from build123d import *

# Parameters (mm, degrees)
PAD_DEPTH       = 40
POCKET_DEPTH    = 35
FILLET_R        = 2
SKETCH002_R     = 1.75
POCKET001_DEPTH = 40.001


with BuildPart() as part:
    # Sketch → Pad (new body)
    with BuildSketch(Plane.XY):
        with BuildLine():
            ThreePointArc((14.201108, 23.840953), (-0.00078, 27.75), (-14.202448, 23.840154))
            ThreePointArc((-14.202448, 23.840154), (-14.967616, 21.462867), (-13.949732, 19.182322))
            ThreePointArc((-19.182322, 13.949732), (-13.949732, 13.949732), (-13.949732, 19.182322))
            ThreePointArc((-19.182322, 13.949732), (-21.992232, 14.881289), (-24.417911, 13.184389))
            ThreePointArc((-24.417911, 13.184389), (-27.743827, -0.585306), (-23.840136, -14.202479))
            ThreePointArc((-23.840136, -14.202479), (-21.462853, -14.967618), (-19.182322, -13.949732))
            ThreePointArc((-13.949732, -13.949732), (-16.566027, -12.866027), (-19.182322, -13.949732))
            ThreePointArc((-13.949732, -13.949732), (0, -19.7279), (13.949732, -13.949732))
            ThreePointArc((19.182322, -13.949732), (16.566027, -12.866027), (13.949732, -13.949732))
            ThreePointArc((19.182322, -13.949732), (21.462854, -14.967618), (23.840137, -14.202477))
            ThreePointArc((23.840137, -14.202477), (27.75, -4.3e-05), (23.840181, 14.202403))
            ThreePointArc((23.840181, 14.202403), (21.462879, 14.967595), (19.182307, 13.949717))
            ThreePointArc((13.934503, 19.167004), (13.957373, 13.942113), (19.182307, 13.949717))
            ThreePointArc((13.934503, 19.167004), (14.950896, 21.453606), (14.201108, 23.840953))
        make_face()
    extrude(amount=PAD_DEPTH)

    # Sketch001 (on Face15 of Pad) → Pocket (cut)
    with BuildSketch(Plane(origin=(0, 0, 0), x_dir=(1, 0, 0), z_dir=(0, 0, -1))):
        with BuildLine():
            ThreePointArc((-21.578938, 12.120723), (-16.766795, 9.869036), (-11.828409, 11.828414))
            ThreePointArc((11.828412, 11.828411), (2e-06, 16.7279), (-11.828409, 11.828414))
            ThreePointArc((11.828412, 11.828411), (16.766797, 9.869036), (21.578938, 12.120723))
            ThreePointArc((21.578938, -12.120723), (24.75, 0), (21.578938, 12.120723))
            ThreePointArc((21.578938, -12.120723), (11.828412, -11.828412), (12.120723, -21.578938))
            ThreePointArc((-12.120723, -21.578938), (0, -24.75), (12.120723, -21.578938))
            ThreePointArc((-12.120723, -21.578938), (-11.828412, -11.828412), (-21.578938, -12.120723))
            ThreePointArc((-21.578938, 12.120723), (-24.75, 0), (-21.578938, -12.120723))
        make_face()
    extrude(amount=-POCKET_DEPTH, mode=Mode.SUBTRACT)

    # Fillet
    fillet_edges = [part.edges().sort_by_distance(p)[0] for p in [
        (-21.578938, 12.120723, 17.5),
        (-12.120723, 21.578938, 17.5),
        (12.120723, 21.578938, 17.5),
        (21.578938, 12.120723, 17.5),
        (21.578938, -12.120723, 17.5),
        (-21.578938, -12.120723, 17.5),
    ]]
    fillet(fillet_edges, radius=FILLET_R)

    # Sketch002 (on Face31 of Fillet) → Pocket001 (cut, through all)
    with BuildSketch(Plane.XY.offset(40)):
        Circle(SKETCH002_R)
    extrude(amount=-POCKET001_DEPTH, mode=Mode.SUBTRACT)


solid = part.part
CAD build for the part. Positions are in the model's coordinates, mm. A direction names the side the tool comes from. Round coordinates to 2 decimals unless told otherwise and drop trailing zeros. Write each loop counter-clockwise with the first axis right and the second up, starting at its lowest first coordinate (ties: lowest second). Pieces come first, ordered by that corner, then holes. Notation, with made-up numbers: M 87.5,60.25 L 127.5,60.25 A5 ccw 127.5,66.25 Z; hole C -7.5,-16 d6. An arc over 180 degrees is marked long. Use a Markdown table: item, result. Add a question column.
1. Slice it at C-C on x = 17. Give the cut face in (y, z).
2. Pull direction X, two halves, no side cores. Call faces 3 (the face through (-10.4, 14.7, 0)), 4 (the face through (13.9, 14, 19.7)), 5 (the face through (-27.747, -0.385, 19.72)): released by +X, released by -X, zero draft, split by the parting line, or undercut.
3. Slice it at B-B on x = 0. Give the cut face in (y, z), then the cut area to 3 significant figures.
4. Drill centre lines: probe 1 along Y at (x, z) = (0, 36.6); probe 2 along Y at (x, z) = (4, 5); probe 3 along Z at (x, y) = (5.5, 13.5). Where is each one in solid material? Low to high.
5. Flat gauge pins, fed straight in: P1, Ø2, axis at y = -8.5, z = 5, coming from the -X side; P2, Ø1.5, axis at x = 18.5, y = -1, coming from the -Z side; P3, Ø8, axis at x = 7.5, z = 15, coming from the -Y side. Where does each tip first touch, or does it go through?
6. 3-axis set-ups, long thin cutter, end or side, ignore diameter. For faces 1 (the face through (11.92, 11.74, 17.26)), 2 (the face through (-0.217, -19.727, 19.72)): which of +Z, -Z, +X, -X, +Y, -Y reach the whole face in a straight line?
7. Slice it at A-A on y = 0. Give the cut face in (x, z).
Reply:
| question | item | result |
|---|---|---|
| 1 | outline | M -12.89,0 L -9.88,0 L -9.88,35 L 9.88,35 L 9.88,0 L 12.89,0 L 12.89,40 L -12.89,40 Z |
| 2 | face 3 | zero draft |
| 2 | face 4 | undercut |
| 2 | face 5 | released by -X |
| 3 | outline | M -19.73,0 L -16.73,0 L -16.73,35 L -1.75,35 L -1.75,40 L -19.73,40 Z; M 1.75,35 L 24.75,35 L 24.75,0 L 27.75,0 L 27.75,40 L 1.75,40 Z |
| 3 | area | 430 mm^2 |
| 4 | probe 1 | y = -19.73 to -1.75, 1.75 to 27.75 |
| 4 | probe 2 | y = -19.32 to -16.24, 24.42 to 27.46 |
| 4 | probe 3 | z = 35 to 40 |
| 5 | P1 | stops at x = -26.72 |
| 5 | P2 | stops at z = 35 |
| 5 | P3 | stops at y = -19.41 |
| 6 | face 1 | -Z |
| 6 | face 2 | +Z, -Z, -Y |
| 7 | outline | M -27.75,0 L -24.75,0 L -24.75,35 L -1.75,35 L -1.75,40 L -27.75,40 Z; M 1.75,35 L 24.75,35 L 24.75,0 L 27.75,0 L 27.75,40 L 1.75,40 Z |
